Read the model definition and answer for the solid it produces. Units are mm, in the model's axes. Face numbers are marked on the shaded views. Give positions to 0.01 mm unless a question says otherwise; leave off trailing zeros. Order: outer loops, then holes, each group sorted by start corner. A loop starts at its lowest first (then second) coordinate and runs counter-clockwise, first axis right, second up. Notation, with made-up numbers: (19, 26) - (62, 26) arc R27 ccw to (62, 55) - close; hole circle Ø8 at (79.25, 30.5). An arc over 180 degrees is marked (long way). Write item = value, one per line.
```python
from build123d import *

# Parameters (mm, degrees)
ALUM_C_CHNL_SHORT_BOSS_EXTRUDE3_DEPTH      = 254
ALUM_C_CHNL_SHORT_BOSS_EXTRUDE3_DEPTH_BACK = 254
SKETCH12_R                                 = 3.25
CUT_EXTRUDE9_DEPTH                         = 3.175
SKETCH8_R                                  = 3.25
CUT_EXTRUDE5_DEPTH                         = 20
LPATTERN4_COUNT                            = 25
LPATTERN4_PITCH                            = 10
LPATTERN3_COUNT                            = 25
LPATTERN3_PITCH                            = 10


with BuildPart() as part:
    # Sketch3 → Alum C chnl SHORT Boss-Extrude3 (new body, two sides)
    with BuildSketch(Plane(origin=(0, 0, 0), x_dir=(0, 0, -1), z_dir=(1, 0, 0))) as alum_c_chnl_short_boss_extrude3_sk:
        Polygon((-304.8, 12.7), (-254, 12.7), (-254, 114.3), (-304.8, 114.3), (-304.8, 111.125), (-257.175, 111.125), (-257.175, 15.875), (-304.8, 15.875), align=None)
    extrude(amount=ALUM_C_CHNL_SHORT_BOSS_EXTRUDE3_DEPTH)
    extrude(alum_c_chnl_short_boss_extrude3_sk.sketch, amount=-ALUM_C_CHNL_SHORT_BOSS_EXTRUDE3_DEPTH_BACK)

    # Sketch12 → Cut-Extrude9 (cut)
    with BuildSketch(Plane(origin=(0, 15.875, 0), x_dir=(1, 0, 0), z_dir=(0, 1, 0))):
        with Locations((-225, -285)):
            Circle(SKETCH12_R)
        with Locations((0, -285)):
            Circle(SKETCH12_R)
        with Locations((225, -285)):
            Circle(SKETCH12_R)
    extrude(amount=-CUT_EXTRUDE9_DEPTH, mode=Mode.SUBTRACT)

    # Sketch8 → Cut-Extrude5 (cut)
    with BuildSketch(Plane(origin=(0, 114.3, 0), x_dir=(1, 0, 0), z_dir=(0, 1, 0))):
        with Locations((0, -280.2)):
            Circle(SKETCH8_R)
    cut_extrude5 = extrude(amount=-CUT_EXTRUDE5_DEPTH, mode=Mode.SUBTRACT)

    # LPattern4: Cut-Extrude5 ×25
    with Locations(*[(-i * LPATTERN4_PITCH, 0, 0) for i in range(1, LPATTERN4_COUNT)]):
        add(cut_extrude5, mode=Mode.SUBTRACT)

    # LPattern3: Cut-Extrude5 ×25
    with Locations(*[(i * LPATTERN3_PITCH, 0, 0) for i in range(1, LPATTERN3_COUNT)]):
        add(cut_extrude5, mode=Mode.SUBTRACT)


solid = part.part
```
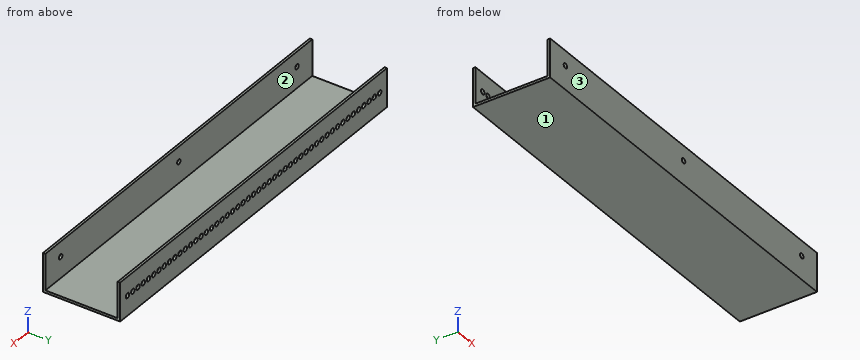
1. Straight lines are drawn through the part: L1, parallel to Y at x = -133, z = 258.5 (3 decimals); L2, parallel to Z at x = 180, y = 112.85; L3, parallel to Z at x = 0, y = 14. For each, find the intervals that lie inside material, in ascending order. Write a range as [from, to].
Recorded:
L1 = [12.7, 15.875], [111.125, 114.3]
L2 = [254, 276.95], [283.45, 304.8]
L3 = [254, 281.75], [288.25, 304.8]
2. Section B-B (y = 96) is taken. Determine the outline of the cut face in (x, z) (3 decimals).
Recorded:
outline = (-254, 254) - (254, 254) - (254, 257.175) - (-254, 257.175) - close
3. Section A-A (z = 264.5) is taken. Determine the outline of the cut face in (x, y) (3 decimals), and give its area (3 significant figures).
Recorded:
outline = (-254, 12.7) - (254, 12.7) - (254, 15.875) - (-254, 15.875) - close; (-254, 111.125) - (254, 111.125) - (254, 114.3) - (-254, 114.3) - close
area = 3,230 mm^2
4. A flat-ended cylindrical pin translates along its axis: pin 1 (6 mm diameter, centred on x = -90, z = 280.2, fed in from +Y) (3 decimals). Find the tip coordinate at first contact, or state that the pin passes through.
Recorded:
pin_1 = 15.875
5. Determine the mould class of the marked faces 1, 2 and 3 for opening direction Y: +Y half, -Y half, draft (parallel to the pull), parting line (faces both ways), or undercut.
Recorded:
face_1 = draft
face_2 = undercut
face_3 = -Y half
